```python
from build123d import *

# Parameters (mm, degrees)
SKETCH2_R   = 3.2
SKETCH4_W   = 12
SKETCH4_H   = 6.65
SKETCH4_W_2 = 13.7
SKETCH4_H_2 = 10


with BuildPart() as part:
    # Sweep1: sweep along a path in Sketch1
    with BuildLine(Plane.XY) as sweep1_path:
        ThreePointArc((0, 0), (8.491378029, 20.5), (28.991378029, 28.991378029))
    # Sketch2 → Sweep1 (sweep)
    with BuildSketch(Plane(origin=(0, 0, 0), x_dir=(1, 0, 0), z_dir=(0, 1, 0))):
        Circle(SKETCH2_R)
    sweep(path=sweep1_path.line)

    # Sketch4 → Revolve1 (revolve)
    with BuildSketch(Plane.XY, mode=Mode.PRIVATE) as revolve1_sk:
        with Locations((34.991378029, 32.316378029)):
            Rectangle(SKETCH4_W, SKETCH4_H)
        Polygon((55.123871223, 28.991378029), (40.991378029, 28.991378029), (40.991378029, 35.641378029), (45.123871223, 39.991378029), (55.123871223, 39.991378029), align=None)
        Polygon((73.231001973, 28.991378029), (55.123871223, 28.991378029), (55.123871223, 39.991378029), (57.231001973, 43.391378029), (57.231001973, 44.891378029), (73.231001973, 44.891378029), align=None)
        with Locations((80.081001973, 33.991378029)):
            Rectangle(SKETCH4_W_2, SKETCH4_H_2)
    revolve(revolve1_sk.sketch.rotate(Axis((28.991378029, 28.991378029, 0), (1, 0, 0)), 90), axis=Axis((28.991378029, 28.991378029, 0), (1, 0, 0)))  # turned: the seam where the file's is


solid = part.part
```
Geometry: final body of the model. Coordinates: model frame, mm. Coordinates: 2 decimals unless noted, no trailing zeros. Order: outer loops, then holes, each group sorted by start corner. A loop starts at its lowest first (then second) coordinate and runs counter-clockwise, first axis right, second up. Notation, with made-up numbers: (25.5, 48) - (69.5, 48) arc R23 cw to (69.5, 78) - close; hole circle Ø7 at (52.5, 65.25). An arc over 180 degrees is marked (long way). Return JSON: item names as keys, results as strings. Group by question number.
1. Cut plane B-B (z = 0). Output: boundary loops of the cut face in (x, y).
2. Pull-direction query (X, two-part tool) for faces 1 (the face through (73.231, 39.4, -0.2)), 2 (the face through (80.177, 37.863, 4.614)), 3 (the face through (28.991, 27, -3)); classes: pulls with the +X half, pulls with the -X half, needs draft (parallel to the pull), parting line crosses it, or undercut.
3. Material intervals for line 1 along X through (y, z) = (28, 5.5); line 2 along X through (y, z) = (19.5, 0.5); line 3 along Y through (x, z) = (69.5, 0), sorted ascending. Write a range as [from, to].
4. Cut plane A-A (x = 79). Output: boundary loops of the cut face in (y, z), plus the area to 3 significant figures.
5. Pin query (flat end, axial travel): pin 1 (3 mm diameter, centred on y = 22.5, z = -10, fed in from +X); pin 2 (2 mm diameter, centred on x = 56.5, y = 37, fed in from +Z); pin 3 (6 mm diameter, centred on x = 34.5, z = -1, fed in from -Y). Return the tip coordinate at first contact, or that it passes through.
6. Cut plane C-C (x = 39.5). Output: boundary loops of the cut face in (y, z), plus the area to 3 significant figures.
Resolved:
{
 "1": {"outline": "(-3.2, 0) - (3.2, 0) arc R25.79 cw to (28.99, 25.79) - (28.99, 22.34) - (40.99, 22.34) - (45.12, 17.99) - (55.12, 17.99) - (57.23, 14.59) - (57.23, 13.09) - (73.23, 13.09) - (73.23, 18.99) - (86.93, 18.99) - (86.93, 38.99) - (73.23, 38.99) - (73.23, 44.89) - (57.23, 44.89) - (57.23, 43.39) - (55.12, 39.99) - (45.12, 39.99) - (40.99, 35.64) - (28.99, 35.64) - (28.99, 32.19) arc R32.19 ccw to start"},
 "2": {"face 1": "pulls with the +X half", "face 2": "needs draft", "face 3": "undercut"},
 "3": {"line 1": "x = [28.99, 86.93]", "line 2": "x = [3.43, 12.05], [43.7, 86.93]", "line 3": "y = [13.09, 44.89]"},
 "4": {"outline": "circle Ø20 at (28.99, 0)", "area": "314 mm²"},
 "5": {"pin 1": "stops at x = 73.23", "pin 2": "stops at z = 14.11", "pin 3": "stops at y = 22.34"},
 "6": {"outline": "circle Ø13.3 at (28.99, 0)", "area": "139 mm²"}
}
